from build123d import *

# Parameters (mm, degrees)
SKETCH4_W           = 31.75
SKETCH4_H           = 19.75
BOSS_EXTRUDE1_DEPTH = 19
SHELL1_T            = 2
SKETCH5_W           = 12
SKETCH5_H           = 20.5
CUT_EXTRUDE1_DEPTH  = 2


with BuildPart() as part:
    # Sketch4 → Boss-Extrude1 (new body)
    with BuildSketch(Plane(origin=(0, 0, 0), x_dir=(0, 0, -1), z_dir=(1, 0, 0))):
        Rectangle(SKETCH4_W, SKETCH4_H)
    extrude(amount=BOSS_EXTRUDE1_DEPTH)

    # Shell1
    shell1_openings = [part.faces().sort_by_distance(p)[0] for p in [
        (0, 0, 0),
    ]]
    offset(amount=SHELL1_T, openings=shell1_openings, kind=Kind.INTERSECTION)

    # Sketch5 → Cut-Extrude1 (cut)
    with BuildSketch(Plane(origin=(0, 11.875, 0), x_dir=(1, 0, 0), z_dir=(0, 1, 0))):
        with Locations((6, 5.625)):
            Rectangle(SKETCH5_W, SKETCH5_H)
    extrude(amount=-CUT_EXTRUDE1_DEPTH, mode=Mode.SUBTRACT)


solid = part.part
For this review, take the finished solid that the model builds, in its own axes (mm). A direction names the side the tool comes from. Coordinates: 2 decimals unless noted, no trailing zeros. Write each loop counter-clockwise with the first axis right and the second up, starting at its lowest first coordinate (ties: lowest second). Pieces come first, ordered by that corner, then holes. Notation, with made-up numbers: (41, 68.5) -> (84, 68.5) arc R20 ccw to (84, 98.5) -> close; hole circle Ø9 at (14.5, 8.5). An arc over 180 degrees is marked (long way). Write each question's results on one line, items separated by ' | '. Start each with the question number.
1) Consider section A-A (y = -5.75). Write out the cut boundary in (x, z) (3 decimals).
2) Consider section C-C (z = 0.5). Write out the cut boundary in (x, y) (3 decimals).
3) Wall thickness on L1, parallel to Z at x = 11.5, y = -6 (3 decimals); L2, parallel to Y at x = 2.25, z = 13 (3 decimals); L3, parallel to Z at x = 3, y = 10.75 (3 decimals): over which ranges is each line inside the solid? List them lowest first. Write a range as [from, to].
4) Insertion check: pin 1 (0.6 mm diameter, centred on y = 11, z = -9, fed in from -X); pin 2 (10 mm diameter, centred on y = 1.5, z = -4.5, fed in from -X). Each pin has a flat end and moves straight along its axis. Give the tip position at first contact, or say it passes through.
5) The part is to be moulded in two halves that separate along Z. For faces 1 (the face through (10, 0, 17.875)), 2 (the face through (10, -11.875, 0)), 3 (the face through (6, 11, 4.625)), 4 (the face through (9, 0, 15.875)), say which applies: +Z half, -Z half, draft (parallel to the pull), parting line (faces both ways), or undercut.
6) Consider section B-B (x = 14.25). Write out the cut boundary in (y, z) (3 decimals).
7) For faces 5 (the face through (12, 11, -5)), 6 (the face through (19, 0, 0)), 7 (the face through (21, 0, 0)), list the 3-axis set-ups (+Z, -Z, +X, -X, +Y, -Y) from which the entire face can be reached by the end or side of a thin tool; tool diameter is ignored.
8) Consider section D-D (x = 4.5). Write out the cut boundary in (y, z) (3 decimals), plus the area to 3 significant figures.
Geometry says:
1) outline: (0, -17.875) -> (21, -17.875) -> (21, 17.875) -> (0, 17.875) -> (0, 15.875) -> (19, 15.875) -> (19, -15.875) -> (0, -15.875) -> close
2) outline: (0, -11.875) -> (21, -11.875) -> (21, 11.875) -> (12, 11.875) -> (12, 9.875) -> (19, 9.875) -> (19, -9.875) -> (0, -9.875) -> close
3) L1: [-17.875, -15.875], [15.875, 17.875] | L2: [-11.875, -9.875], [9.875, 11.875] | L3: [-17.875, -15.875], [4.625, 17.875]
4) pin 1: x = 12 | pin 2: x = 19
5) face 1: +Z half | face 2: draft | face 3: undercut | face 4: undercut
6) outline: (-11.875, -17.875) -> (11.875, -17.875) -> (11.875, 17.875) -> (-11.875, 17.875) -> close; hole (-9.875, -15.875) -> (9.875, -15.875) -> (9.875, 15.875) -> (-9.875, 15.875) -> close
7) face 5: -X, +Y | face 6: -X | face 7: +Z, -Z, +X, +Y, -Y
8) outline: (-11.875, -17.875) -> (11.875, -17.875) -> (11.875, -15.875) -> (-9.875, -15.875) -> (-9.875, 15.875) -> (9.875, 15.875) -> (9.875, 4.625) -> (11.875, 4.625) -> (11.875, 17.875) -> (-11.875, 17.875) -> close | area: 181 mm^2
